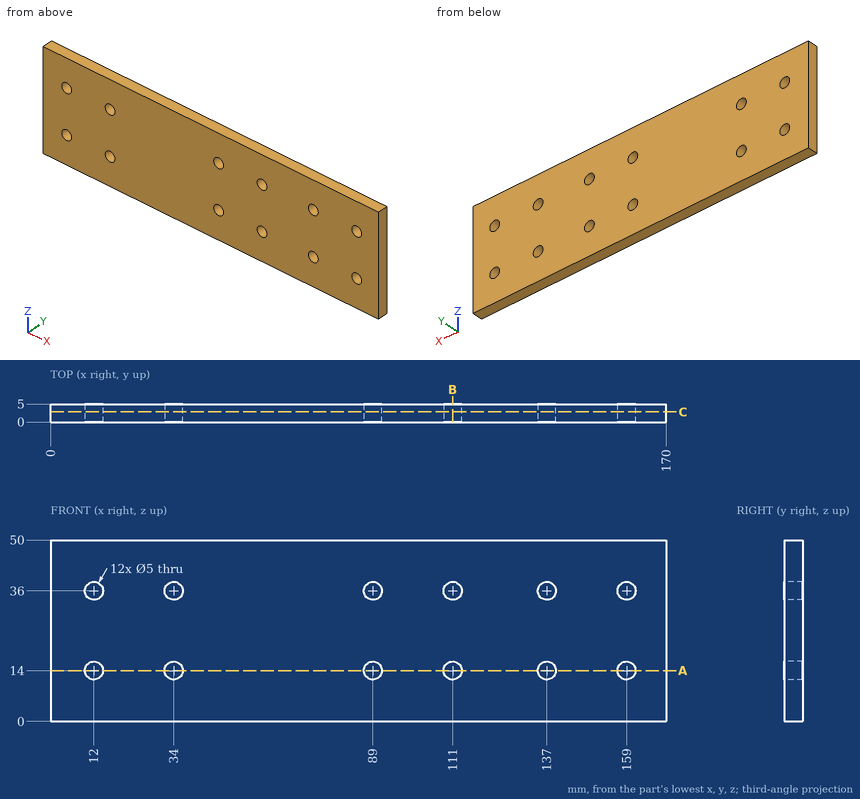
Check sheet for the drawn part. Datum: minimum x, y, z corner. Units: mm. Coordinates: 2 decimals unless noted, no trailing zeros. Order: outer loops, then holes, each group sorted by start corner. A loop starts at its lowest first (then second) coordinate and runs counter-clockwise, first axis right, second up. Notation, with made-up numbers: (49, 58.5) -> (104, 58.5) arc R35 ccw to (104, 91.5) -> close; hole circle Ø10 at (6, 11). An arc over 180 degrees is marked (long way). Use a Markdown table: item, result. Add a question column.
1. Cross-section at B-B (x = 111). Enter the section's corners in (y, z).
2. Cross-section at C-C (y = 2.8). Give the number of separate pieces and of enclosed holes in the cut face, and give its area (3 significant figures).
3. Cross-section at A-A (z = 14). Enter the section's corners in (x, y), and give its area (3 significant figures).
4. Material ranges on L1, parallel to Z at x = 137, y = 2; L2, parallel to Z at x = 110.5, y = 0.4, recorded low to high.
Filled sheet:
| question | item | result |
|---|---|---|
| 1 | outline | (0, 0) -> (5, 0) -> (5, 11.5) -> (0, 11.5) -> close; (0, 16.5) -> (5, 16.5) -> (5, 33.5) -> (0, 33.5) -> close; (0, 38.5) -> (5, 38.5) -> (5, 50) -> (0, 50) -> close |
| 2 | separate pieces | 1 |
| 2 | enclosed holes | 12 |
| 2 | area | 8,260 mm2 |
| 3 | outline | (0, 0) -> (9.5, 0) -> (9.5, 5) -> (0, 5) -> close; (14.5, 0) -> (31.5, 0) -> (31.5, 5) -> (14.5, 5) -> close; (36.5, 0) -> (86.5, 0) -> (86.5, 5) -> (36.5, 5) -> close; (91.5, 0) -> (108.5, 0) -> (108.5, 5) -> (91.5, 5) -> close; (113.5, 0) -> (134.5, 0) -> (134.5, 5) -> (113.5, 5) -> close; (139.5, 0) -> (156.5, 0) -> (156.5, 5) -> (139.5, 5) -> close; (161.5, 0) -> (170, 0) -> (170, 5) -> (161.5, 5) -> close |
| 3 | area | 700 mm2 |
| 4 | L1 | 0 to 11.5, 16.5 to 33.5, 38.5 to 50 |
| 4 | L2 | 0 to 11.55, 16.45 to 33.55, 38.45 to 50 |
